Here's how the part is built. I have some questions about the finished solid (model axes, mm). Face numbers are marked on the shaded views. A direction names the side the tool comes from. Round coordinates to 2 decimals unless told otherwise and drop trailing zeros. Write each loop counter-clockwise with the first axis right and the second up, starting at its lowest first coordinate (ties: lowest second). Pieces come first, ordered by that corner, then holes. Notation, with made-up numbers: (77, 6) - (114, 6) arc R31 ccw to (114, 45) - close; hole circle Ø3 at (-1.5, 2). An arc over 180 degrees is marked (long way). Write item = value, one per line. Start each with the question number.
Item 1: If we section it at A-A (z = 1.75): Give the number of separate pieces and of enclosed holes in the cut face, and give its area (3 significant figures).
Item 2: Which directions (+Z, -Z, +X, -X, +Y, -Y) give clear straight access to the entire face, cutting with the end or side of a thin tool? Please do the marked faces 4 and 5.
Item 3: If we section it at B-B (y = 0): Please give me the cut outline in (x, z), and give its area (3 significant figures).
Item 4: For P1, Ø1, axis at x = 1, y = -0.5, coming from the +Z side; P2, Ø0.7, axis at y = 3.5, z = -2, coming from the +X side; P3, Ø2, axis at x = 0.5, z = -4, coming from the -Y side, each with a flat end and sliding along its axis, tell me the tip position at first contact or that it passes through.
Item 5: If I drill on line 1 along X through (y, z) = (3.75, -0.75); line 2 along Y through (x, z) = (-4, 2.25) (3 decimals); line 3 along Z through (x, y) = (-4, -3), over which ranges is the centre line in solid material (lowest first)? Write a range as [from, to].
Item 6: Thinking about a two-plate mould opening in Y: for the marked faces 1, 2 and 3, which applies, pulls with the +Y half, pulls with the -Y half, needs draft (parallel to the pull), parting line crosses it, or undercut?
Item 7: If we section it at C-C (x = 0.25): Please give me the cut outline in (y, z).
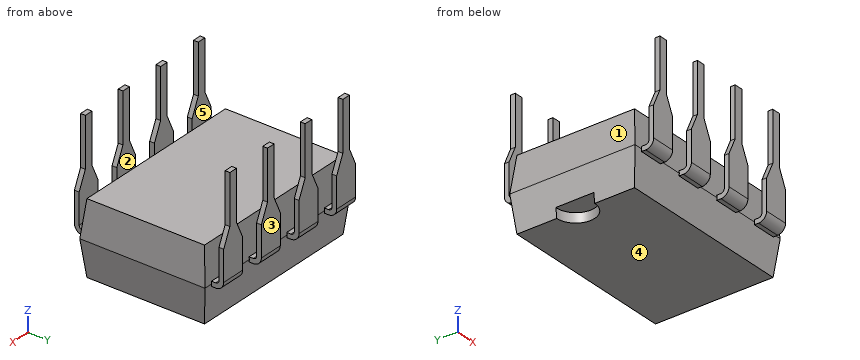
```python
from build123d import *

# Parameters (mm, degrees)
RESSALTO_EXTRUS_O1_DEPTH        = 4.9
CORTE_EXTRUS_O2_DEPTH           = 3.55
ESBO_O8_R                       = 1
CORTE_EXTRUS_O5_DEPTH           = 0.5
ESBO_O6_W                       = 1.275
ESBO_O6_H                       = 0.25
RESSALTO_EXTRUS_O2_DEPTH        = 0.025
ESBO_O7_W                       = 1.275
ESBO_O7_H                       = 0.25
CORTE_EXTRUS_O6_START           = -0.25
CORTE_EXTRUS_O6_DEPTH           = 0.25
ESBO_O10_W                      = 0.445
ESBO_O10_H                      = 0.25
RESSALTO_EXTRUS_O3_DEPTH        = 2.6
PADR_O_LINEAR1_COUNT            = 4
PADR_O_LINEAR1_PITCH            = 2.54
PADR_O_LINEAR1_COPY_1_SKETCH_W  = 1.275
PADR_O_LINEAR1_COPY_1_SKETCH_H  = 0.25
PADR_O_LINEAR1_COPY_1_DEPTH     = 0.025
PADR_O_LINEAR1_COPY_2_SKETCH_W  = 1.275
PADR_O_LINEAR1_COPY_2_SKETCH_H  = 0.25
PADR_O_LINEAR1_COPY_2_DEPTH     = 0.025
PADR_O_LINEAR1_COPY_3_SKETCH_W  = 1.275
PADR_O_LINEAR1_COPY_3_SKETCH_H  = 0.25
PADR_O_LINEAR1_COPY_3_DEPTH     = 0.025
PADR_O_LINEAR1_COPY_4_SKETCH_W  = 1.275
PADR_O_LINEAR1_COPY_4_SKETCH_H  = 0.25
PADR_O_LINEAR1_COPY_5_SKETCH_W  = 1.275
PADR_O_LINEAR1_COPY_5_SKETCH_H  = 0.25
PADR_O_LINEAR1_COPY_6_SKETCH_W  = 1.275
PADR_O_LINEAR1_COPY_6_SKETCH_H  = 0.25
PADR_O_START                    = -0.25
PADR_O_LINEAR1_COPY_7_DEPTH     = 0.25
PADR_O_LINEAR1_COPY_8_DEPTH     = 0.25
PADR_O_LINEAR1_COPY_9_DEPTH     = 0.25
PADR_O_LINEAR1_COPY_10_SKETCH_W = 0.445
PADR_O_LINEAR1_COPY_10_SKETCH_H = 0.25
PADR_O_LINEAR1_COPY_10_DEPTH    = 2.6
PADR_O_LINEAR1_COPY_11_SKETCH_W = 0.445
PADR_O_LINEAR1_COPY_11_SKETCH_H = 0.25
PADR_O_LINEAR1_COPY_11_DEPTH    = 2.6
PADR_O_LINEAR1_COPY_12_SKETCH_W = 0.445
PADR_O_LINEAR1_COPY_12_SKETCH_H = 0.25
PADR_O_LINEAR1_COPY_12_DEPTH    = 2.6


with BuildPart() as part:
    # Esboço1 → Ressalto-extrusão1 (new, symmetric)
    with BuildSketch(Plane(origin=(0, 0, 0), x_dir=(0, 0, -1), z_dir=(1, 0, 0))):
        Polygon((0.9, 3.1), (0.9, -3.1), (2.8, -3.3), (4.7, -3.1), (4.7, 3.1), (2.8, 3.3), align=None)
    extrude(amount=RESSALTO_EXTRUS_O1_DEPTH, both=True)

    # Esboço3 → Corte-extrusão2 (cut, symmetric)
    with BuildSketch(Plane(origin=(0, 0, 0), x_dir=(1, 0, 0), z_dir=(0, 1, 0))):
        Polygon((-4.9, 2.8), (-4.669897634, 4.726835982), (-5.836348907, 4.726835982), (-5.836348907, 0.873164018), (-4.669897634, 0.873164018), align=None)
    corte_extrus_o2 = extrude(amount=CORTE_EXTRUS_O2_DEPTH, both=True, mode=Mode.SUBTRACT)

    # Espelhar1: Corte-extrusão2 across plane
    add(corte_extrus_o2.mirror(Plane(origin=(0, 0, 0), x_dir=(0, 0, 1), z_dir=(1, 0, 0))), mode=Mode.SUBTRACT)

    # Esboço8 → Corte-extrusão5 (cut)
    with BuildSketch(Plane(origin=(0, 0, -4.7), x_dir=(-1, 0, 0), z_dir=(0, 0, -1))):
        with Locations((4.673102382, 0)):
            Circle(ESBO_O8_R)
    extrude(amount=-CORTE_EXTRUS_O5_DEPTH, mode=Mode.SUBTRACT)

    # Esboço6 → Ressalto-extrusão2 (add, symmetric)
    with BuildSketch(Plane(origin=(0, 3.3, 0), x_dir=(1, 0, 0), z_dir=(0, 1, 0))):
        with Locations((-3.81, 2.8)):
            Rectangle(ESBO_O6_W, ESBO_O6_H)
    ressalto_extrus_o2 = extrude(amount=RESSALTO_EXTRUS_O2_DEPTH, both=True)

    # Varredura1: sweep along a curve in space
    with BuildLine() as varredura1_path:
        Line((-3.81, 3.325, -2.8), (-3.81, 3.51, -2.8))
        ThreePointArc((-3.81, 3.51, -2.8), (-3.81, 3.722132034, -2.712132034), (-3.81, 3.81, -2.5))
        Line((-3.81, 3.81, -2.5), (-3.81, 3.81, 0))
    # Esboço7 → Varredura1 (sweep)
    with BuildSketch(Plane(origin=(0, 3.325, 0), x_dir=(1, 0, 0), z_dir=(0, 1, 0))):
        with Locations((-3.81, 2.8)):
            Rectangle(ESBO_O7_W, ESBO_O7_H)
    varredura1 = sweep(path=varredura1_path.line)

    # Esboço9 → Corte-extrusão6 (cut)
    with BuildSketch(Plane(origin=(0, 3.935, 0), x_dir=(1, 0, 0), z_dir=(0, 1, 0)).offset(CORTE_EXTRUS_O6_START)):
        Polygon((-4.0325, 0), (-4.4475, 0.9), (-4.4475, -0.2), (-3.1725, -0.2), (-3.1725, 0.9), (-3.5875, 0), align=None)
    corte_extrus_o6 = extrude(amount=CORTE_EXTRUS_O6_DEPTH, mode=Mode.SUBTRACT)

    # Esboço10 → Ressalto-extrusão3 (add)
    with BuildSketch(Plane.XY):
        with Locations((-3.81, 3.81)):
            Rectangle(ESBO_O10_W, ESBO_O10_H)
    ressalto_extrus_o3 = extrude(amount=RESSALTO_EXTRUS_O3_DEPTH)

    # Espelhar2: Ressalto-extrusão2, Varredura1, Corte-extrusão6, Ressalto-extrusão3 across plane
    add(ressalto_extrus_o2.mirror(Plane.ZX))
    add(varredura1.mirror(Plane.ZX))
    add(corte_extrus_o6.mirror(Plane.ZX), mode=Mode.SUBTRACT)
    add(ressalto_extrus_o3.mirror(Plane.ZX))

    # Padrão linear1: Ressalto-extrusão2, Varredura1, Corte-extrusão6, Ressalto-extrusão3 ×4
    with Locations(*[(i * PADR_O_LINEAR1_PITCH, 0, 0) for i in range(1, PADR_O_LINEAR1_COUNT)]):
        add(ressalto_extrus_o2)
        add(varredura1)
        add(corte_extrus_o6, mode=Mode.SUBTRACT)
        add(ressalto_extrus_o3)

    # Padrão linear1 copy 1 sketch → Padrão linear1 copy 1 (add, symmetric)
    with BuildSketch(Plane(origin=(2.54, -3.3, 0), x_dir=(1, 0, 0), z_dir=(0, -1, 0))):
        with Locations((-3.81, -2.8)):
            Rectangle(PADR_O_LINEAR1_COPY_1_SKETCH_W, PADR_O_LINEAR1_COPY_1_SKETCH_H)
    extrude(amount=PADR_O_LINEAR1_COPY_1_DEPTH, both=True)

    # Padrão linear1 copy 2 sketch → Padrão linear1 copy 2 (add, symmetric)
    with BuildSketch(Plane(origin=(5.08, -3.3, 0), x_dir=(1, 0, 0), z_dir=(0, -1, 0))):
        with Locations((-3.81, -2.8)):
            Rectangle(PADR_O_LINEAR1_COPY_2_SKETCH_W, PADR_O_LINEAR1_COPY_2_SKETCH_H)
    extrude(amount=PADR_O_LINEAR1_COPY_2_DEPTH, both=True)

    # Padrão linear1 copy 3 sketch → Padrão linear1 copy 3 (add, symmetric)
    with BuildSketch(Plane(origin=(7.62, -3.3, 0), x_dir=(1, 0, 0), z_dir=(0, -1, 0))):
        with Locations((-3.81, -2.8)):
            Rectangle(PADR_O_LINEAR1_COPY_3_SKETCH_W, PADR_O_LINEAR1_COPY_3_SKETCH_H)
    extrude(amount=PADR_O_LINEAR1_COPY_3_DEPTH, both=True)

    # Padrão linear1 copy 4: sweep along a curve in space
    with BuildLine() as padr_o_linear1_copy_4_path:
        Line((-1.27, -3.325, -2.8), (-1.27, -3.51, -2.8))
        ThreePointArc((-1.27, -3.51, -2.8), (-1.27, -3.722132034, -2.712132034), (-1.27, -3.81, -2.5))
        Line((-1.27, -3.81, -2.5), (-1.27, -3.81, 0))
    # Padrão linear1 copy 4 sketch → Padrão linear1 copy 4 (sweep)
    with BuildSketch(Plane(origin=(2.54, -3.325, 0), x_dir=(1, 0, 0), z_dir=(0, -1, 0))):
        with Locations((-3.81, -2.8)):
            Rectangle(PADR_O_LINEAR1_COPY_4_SKETCH_W, PADR_O_LINEAR1_COPY_4_SKETCH_H)
    sweep(path=padr_o_linear1_copy_4_path.line)

    # Padrão linear1 copy 5: sweep along a curve in space
    with BuildLine() as padr_o_linear1_copy_5_path:
        Line((1.27, -3.325, -2.8), (1.27, -3.51, -2.8))
        ThreePointArc((1.27, -3.51, -2.8), (1.27, -3.722132034, -2.712132034), (1.27, -3.81, -2.5))
        Line((1.27, -3.81, -2.5), (1.27, -3.81, 0))
    # Padrão linear1 copy 5 sketch → Padrão linear1 copy 5 (sweep)
    with BuildSketch(Plane(origin=(5.08, -3.325, 0), x_dir=(1, 0, 0), z_dir=(0, -1, 0))):
        with Locations((-3.81, -2.8)):
            Rectangle(PADR_O_LINEAR1_COPY_5_SKETCH_W, PADR_O_LINEAR1_COPY_5_SKETCH_H)
    sweep(path=padr_o_linear1_copy_5_path.line)

    # Padrão linear1 copy 6: sweep along a curve in space
    with BuildLine() as padr_o_linear1_copy_6_path:
        Line((3.81, -3.325, -2.8), (3.81, -3.51, -2.8))
        ThreePointArc((3.81, -3.51, -2.8), (3.81, -3.722132034, -2.712132034), (3.81, -3.81, -2.5))
        Line((3.81, -3.81, -2.5), (3.81, -3.81, 0))
    # Padrão linear1 copy 6 sketch → Padrão linear1 copy 6 (sweep)
    with BuildSketch(Plane(origin=(7.62, -3.325, 0), x_dir=(1, 0, 0), z_dir=(0, -1, 0))):
        with Locations((-3.81, -2.8)):
            Rectangle(PADR_O_LINEAR1_COPY_6_SKETCH_W, PADR_O_LINEAR1_COPY_6_SKETCH_H)
    sweep(path=padr_o_linear1_copy_6_path.line)

    # Padrão linear1 copy 7 sketch → Padrão linear1 copy 7 (cut)
    with BuildSketch(Plane(origin=(2.54, -3.935, 0), x_dir=(1, 0, 0), z_dir=(0, -1, 0)).offset(PADR_O_START)):
        Polygon((-4.0325, 0), (-4.4475, -0.9), (-4.4475, 0.2), (-3.1725, 0.2), (-3.1725, -0.9), (-3.5875, 0), align=None)
    extrude(amount=PADR_O_LINEAR1_COPY_7_DEPTH, mode=Mode.SUBTRACT)

    # Padrão linear1 copy 8 sketch → Padrão linear1 copy 8 (cut)
    with BuildSketch(Plane(origin=(5.08, -3.935, 0), x_dir=(1, 0, 0), z_dir=(0, -1, 0)).offset(PADR_O_START)):
        Polygon((-4.0325, 0), (-4.4475, -0.9), (-4.4475, 0.2), (-3.1725, 0.2), (-3.1725, -0.9), (-3.5875, 0), align=None)
    extrude(amount=PADR_O_LINEAR1_COPY_8_DEPTH, mode=Mode.SUBTRACT)

    # Padrão linear1 copy 9 sketch → Padrão linear1 copy 9 (cut)
    with BuildSketch(Plane(origin=(7.62, -3.935, 0), x_dir=(1, 0, 0), z_dir=(0, -1, 0)).offset(PADR_O_START)):
        Polygon((-4.0325, 0), (-4.4475, -0.9), (-4.4475, 0.2), (-3.1725, 0.2), (-3.1725, -0.9), (-3.5875, 0), align=None)
    extrude(amount=PADR_O_LINEAR1_COPY_9_DEPTH, mode=Mode.SUBTRACT)

    # Padrão linear1 copy 10 sketch → Padrão linear1 copy 10 (add)
    with BuildSketch(Plane(origin=(2.54, 0, 0), x_dir=(1, 0, 0), z_dir=(0, 0, 1))):
        with Locations((-3.81, -3.81)):
            Rectangle(PADR_O_LINEAR1_COPY_10_SKETCH_W, PADR_O_LINEAR1_COPY_10_SKETCH_H)
    extrude(amount=PADR_O_LINEAR1_COPY_10_DEPTH)

    # Padrão linear1 copy 11 sketch → Padrão linear1 copy 11 (add)
    with BuildSketch(Plane(origin=(5.08, 0, 0), x_dir=(1, 0, 0), z_dir=(0, 0, 1))):
        with Locations((-3.81, -3.81)):
            Rectangle(PADR_O_LINEAR1_COPY_11_SKETCH_W, PADR_O_LINEAR1_COPY_11_SKETCH_H)
    extrude(amount=PADR_O_LINEAR1_COPY_11_DEPTH)

    # Padrão linear1 copy 12 sketch → Padrão linear1 copy 12 (add)
    with BuildSketch(Plane(origin=(7.62, 0, 0), x_dir=(1, 0, 0), z_dir=(0, 0, 1))):
        with Locations((-3.81, -3.81)):
            Rectangle(PADR_O_LINEAR1_COPY_12_SKETCH_W, PADR_O_LINEAR1_COPY_12_SKETCH_H)
    extrude(amount=PADR_O_LINEAR1_COPY_12_DEPTH)


solid = part.part
```
Reply:
q1.separate_pieces = 8
q1.enclosed_holes = 0
q1.area = 0.890 mm2
q2.face_4 = -Z, +X, -X, +Y, -Y
q2.face_5 = +Z, +X, -X
q3.outline = (-4.9, -2.8) - (-4.73, -4.2) - (-3.67, -4.2) - (-3.67, -4.7) - (4.67, -4.7) - (4.9, -2.8) - (4.67, -0.9) - (-4.67, -0.9) - close
q3.area = 35.9 mm2
q4.P1 = -0.9
q4.P2 = 4.83
q4.P3 = -3.28
q5.line_1 = [-4.38, -3.24], [-1.84, -0.7], [0.7, 1.84], [3.24, 4.38]
q5.line_2 = [-3.935, -3.685], [3.685, 3.935]
q5.line_3 = [-4.7, -0.9]
q6.face_1 = needs draft
q6.face_2 = undercut
q6.face_3 = pulls with the +Y half
q7.outline = (-3.3, -2.8) - (-3.1, -4.7) - (3.1, -4.7) - (3.3, -2.8) - (3.1, -0.9) - (-3.1, -0.9) - close
